Source: CAD feature listing. Evaluate the final solid. Frame: model axes, mm. Face numbers are marked on the shaded views. A direction names the side the tool comes from. Coordinates: 2 decimals unless noted, no trailing zeros. Order: outer loops, then holes, each group sorted by start corner. A loop starts at its lowest first (then second) coordinate and runs counter-clockwise, first axis right, second up. Notation, with made-up numbers: (65, 10) -> (69, 10) arc R17 cw to (69, 31) -> close; hole circle Ø1 at (-2, -35). An arc over 180 degrees is marked (long way). Write item = value, one per line. Start each with the question number.
Item 1: Mould query, pull axis Z, two halves, no side actions, for the marked faces 1 and 2. Classes: released by +Z, released by -Z, zero draft, split by the parting line, or undercut.
Item 2: Ray query, line 1 along Z through (x, y) = (0, -16.25) (3 decimals); line 2 along Z through (x, y) = (44.45, -14) (1 decimal); line 3 along X through (y, z) = (-24, -65). Return the intervals inside material, ascending. Write a range as [from, to].
Item 3: Section query B-B (x = -4.5). Output: boundary loops of the cut face in (y, z), then the cut area to 3 significant figures.
Item 4: Section query A-A (y = -19.75). Count the separate pieces of the cut face and the enclosed holes in it, then the cut area to 3 significant figures.
Item 5: Contact query for flat-ended pins moving along their axis: pin 1 (4 mm diameter, centred on x = 18.5, y = -5.5, fed in from -Z); pin 2 (10 mm diameter, centred on y = -3, z = 11.5, fed in from +X); pin 3 (3 mm diameter, centred on x = 42.5, y = -5.5, fed in from +Z). Output: stop coordinate, or through.
Item 6: Set-up query: the marked faces 3 and 4. Return all of +Z, -Z, +X, -X, +Y, -Y with unobstructed straight access to the full face (end or side cutting, diameter ignored); none if empty.
Item 7: Section query C-C (z = 5). Output: boundary loops of the cut face in (x, y), then the cut area to 3 significant figures.
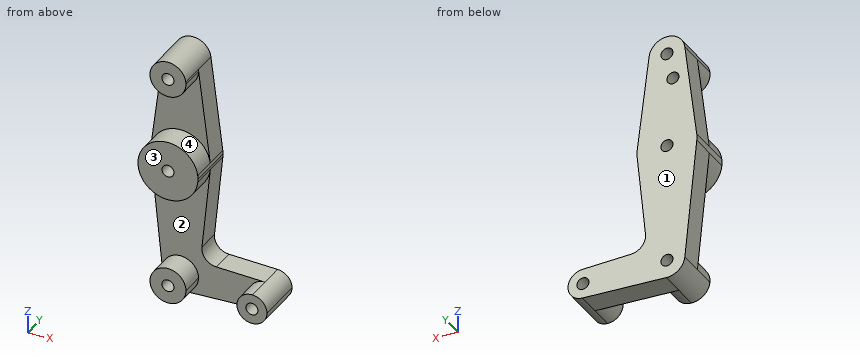
```python
from build123d import *

# Parameters (mm, degrees)
F0_R     = 3.175
F1_DEPTH = 25.4
F2_DEPTH = 12.7


with BuildPart() as f1:
    # F0 (on Front) → F1 (new body)
    with BuildSketch(Plane.XZ):
        with BuildLine():
            ThreePointArc((9.525, 50.8), (9.506305, 51.396483), (9.450293, 51.990625))
            ThreePointArc((9.450293, 51.990625), (0, 60.325), (-9.450293, 51.990625))
            ThreePointArc((-9.450293, 51.990625), (-0.596483, 41.293695), (9.525, 50.8))
        make_face()
        with Locations((0, 50.8)):
            Circle(F0_R, mode=Mode.SUBTRACT)
        with BuildLine():
            ThreePointArc((15.795426, -1.5875), (15.855094, -0.794747), (15.875, 0))
            ThreePointArc((15.875, 0), (15.843841, 0.994139), (15.750488, 1.984375))
            ThreePointArc((15.750488, 1.984375), (0, 15.875), (-15.750488, 1.984375))
            ThreePointArc((-15.750488, 1.984375), (-15.873744, 0.199705), (-15.795426, -1.5875))
            ThreePointArc((-15.795426, -1.5875), (0, -15.875), (15.795426, -1.5875))
        make_face()
        Circle(F0_R, mode=Mode.SUBTRACT)
        with BuildLine():
            ThreePointArc((9.525, -63.5), (-0.476848, -53.986944), (-9.477255, -64.4525))
            ThreePointArc((-9.477255, -64.4525), (-6.262383, -70.67692), (0.340179, -73.018923))
            ThreePointArc((0.340179, -73.018923), (6.854408, -70.113827), (9.525, -63.5))
        make_face()
        with Locations((0, -63.5)):
            Circle(F0_R, mode=Mode.SUBTRACT)
        with BuildLine():
            ThreePointArc((52.3875, -63.5), (50.162007, -57.988477), (44.733482, -55.567564))
            ThreePointArc((44.733482, -55.567564), (36.5125, -63.5), (44.733482, -71.432436))
            ThreePointArc((44.733482, -71.432436), (50.162007, -69.011523), (52.3875, -63.5))
        make_face()
        with Locations((44.45, -63.5)):
            Circle(F0_R, mode=Mode.SUBTRACT)
    extrude(amount=F1_DEPTH)

    # F0 (on Front) → F2 (join)
    with BuildSketch(Plane.XZ):
        with BuildLine():
            ThreePointArc((-15.750488, 1.984375), (0, 15.875), (15.750488, 1.984375))
            Line((15.750488, 1.984375), (9.450293, 51.990625))
            ThreePointArc((9.450293, 51.990625), (9.506305, 51.396483), (9.525, 50.8))
            ThreePointArc((9.525, 50.8), (-0.596483, 41.293695), (-9.450293, 51.990625))
            Line((-9.450293, 51.990625), (-15.750488, 1.984375))
        make_face()
        with Locations((-3.175, 36.5252)):
            Circle(F0_R, mode=Mode.SUBTRACT)
        with BuildLine():
            Line((11.341187, -45.906618), (15.795426, -1.5875))
            ThreePointArc((15.795426, -1.5875), (0, -15.875), (-15.795426, -1.5875))
            Line((-15.795426, -1.5875), (-9.477255, -64.4525))
            ThreePointArc((-9.477255, -64.4525), (-0.476848, -53.986944), (9.525, -63.5))
            ThreePointArc((9.525, -63.5), (6.854408, -70.113827), (0.340179, -73.018923))
            Line((0.340179, -73.018923), (44.733482, -71.432436))
            ThreePointArc((44.733482, -71.432436), (36.5125, -63.5), (44.733482, -55.567564))
            Line((44.733482, -55.567564), (18.9676, -54.646766))
            ThreePointArc((18.9676, -54.646766), (13.2612, -51.928641), (11.341187, -45.906618))
        make_face()
    extrude(amount=F2_DEPTH)


solid = f1.part
```
Computed:
q1.face_1 = zero draft
q1.face_2 = undercut
q2.line_1 = [-73.025, -66.675], [-60.325, -53.975], [-15.875, -3.175], [3.175, 15.875], [41.275, 47.625], [53.975, 60.325]
q2.line_2 = [-71.4, -66.7], [-60.3, -55.6]
q2.line_3 = [-9.41, -2.8], [2.8, 9.41], [36.66, 41.65], [47.25, 52.24]
q3.outline = (-25.4, -71.89) -> (0, -71.89) -> (0, 33.64) -> (-12.7, 33.64) -> (-12.7, 15.22) -> (-25.4, 15.22) -> (-25.4, -15.22) -> (-12.7, -15.22) -> (-12.7, -55.11) -> (-25.4, -55.11) -> close; (-25.4, 42.41) -> (-12.7, 42.41) -> (-12.7, 39.41) -> (0, 39.41) -> (0, 59.19) -> (-25.4, 59.19) -> close
q3.area = 2,400 mm^2
q4.separate_pieces = 4
q4.enclosed_holes = 4
q4.area = 1,430 mm^2
q5.pin_1 = -72.44
q5.pin_2 = 15.18
q5.pin_3 = -55.43
q6.face_3 = +Z, -Z, +X, -X, -Y
q6.face_4 = -Y
q7.outline = (-15.37, -12.7) -> (-15.07, -12.7) -> (-15.07, -25.4) -> (15.07, -25.4) -> (15.07, -12.7) -> (15.37, -12.7) -> (15.37, 0) -> (-15.37, 0) -> close
q7.area = 773 mm^2
